from build123d import *

# Parameters (mm, degrees)
BOSS_EXTRUDE1_DEPTH  = 2
BOSS_EXTRUDE6_DEPTH  = 4.5
CUT_EXTRUDE6_DEPTH   = 4.5
BOSS_EXTRUDE14_DEPTH = 2.3
SKETCH32_R           = 2.1
CUT_EXTRUDE7_DEPTH   = 2.3
SKETCH33_W           = 12.5
SKETCH33_H           = 1.343145751
BOSS_EXTRUDE15_DEPTH = 1.2
SKETCH35_W           = 5.479645997
SKETCH35_H           = 3.827993755
CUT_EXTRUDE8_DEPTH   = 2.4
SKETCH36_W           = 3.7
SKETCH36_H           = 1.827993755
CUT_EXTRUDE9_DEPTH   = 2.4
SKETCH37_R           = 3.9
BOSS_EXTRUDE16_DEPTH = 4.4
CUT_EXTRUDE10_DEPTH  = 7.4
SKETCH43_R           = 2.5
BOSS_EXTRUDE17_DEPTH = 1.2
SKETCH44_R           = 0.95
CUT_EXTRUDE11_DEPTH  = 11
SKETCH45_R           = 2
CUT_EXTRUDE12_DEPTH  = 4.5
SKETCH52_R           = 0.75
CUT_EXTRUDE13_DEPTH  = 10


with BuildPart() as part:
    # Sketch3 → Boss-Extrude1 (new body)
    with BuildSketch(Plane.XY):
        with BuildLine():
            Line((8, 0), (9, -2.5))
            Line((9, -2.5), (9, -7))
            Line((9, -7), (21.5, -7))
            Line((21.5, -7), (25.050252532, -4.949747468))
            ThreePointArc((25.050252532, -4.949747468), (36.467156728, -2.678784027), (30, 7))
            Line((30, 7), (27, 7.5))
            Line((27, 7.5), (5.656854249, 7.5))
            Line((5.656854249, 7.5), (5.656854249, 5.656854249))
            ThreePointArc((5.656854249, 5.656854249), (7.39103626, 3.061467459), (8, 0))
        make_face()
    extrude(amount=BOSS_EXTRUDE1_DEPTH)

    # Sketch22 → Boss-Extrude6 (add)
    with BuildSketch(Plane.XY.offset(2)):
        with BuildLine():
            Line((5.656854249, 5.656854249), (2.486790148, 5.656854249))
            Line((2.486790148, 5.656854249), (2.486790148, 7.5))
            Line((2.486790148, 7.5), (5.656854249, 7.5))
            Line((5.656854249, 7.5), (21.5, 7.5))
            Line((21.5, 7.5), (27, 7.5))
            Line((27, 7.5), (27, 2.172006245))
            Line((27, 2.172006245), (23.275126266, 2.172006245))
            Line((23.275126266, 2.172006245), (23.275126266, -5.974873734))
            Line((23.275126266, -5.974873734), (21.5, -7))
            Line((21.5, -7), (9, -7))
            Line((9, -7), (9, -2.5))
            Line((9, -2.5), (8, 0))
            ThreePointArc((8, 0), (7.39103626, 3.061467459), (5.656854249, 5.656854249))
        make_face()
    extrude(amount=BOSS_EXTRUDE6_DEPTH)

    # Sketch26 → Cut-Extrude6 (cut)
    with BuildSketch(Plane.XY.offset(2)):
        Polygon((18.098080448, 5.3), (2.530052458, 5.3), (2.530052458, 4), (18.098080448, 4), (27, 4), (27, 5.3), align=None)
    extrude(amount=CUT_EXTRUDE6_DEPTH, mode=Mode.SUBTRACT)


with BuildPart() as body_2:
    # Sketch31 → Boss-Extrude14 (new body)
    with BuildSketch(Plane.XY.offset(6.5)):
        with BuildLine():
            Line((2.432688066, 5.656854249), (0, 5.656854249))
            ThreePointArc((0, 5.656854249), (-5.656854249, 0), (0, -5.656854249))
            Line((0, -5.656854249), (9, -5.656854249))
            Line((9, -5.656854249), (9, -7))
            Line((9, -7), (21.5, -7))
            Line((21.5, -7), (23.275126266, -5.974873734))
            Line((23.275126266, -5.974873734), (23.275126266, 2.172006245))
            Line((23.275126266, 2.172006245), (27, 2.172006245))
            Line((27, 2.172006245), (27, 7.5))
            Line((27, 7.5), (2.486790148, 7.5))
            Line((2.486790148, 7.5), (2.432688066, 5.656854249))
        make_face()
    extrude(amount=BOSS_EXTRUDE14_DEPTH)

    # Sketch32 → Cut-Extrude7 (cut)
    with BuildSketch(Plane.XY.offset(8.8)):
        Circle(SKETCH32_R)
    extrude(amount=-CUT_EXTRUDE7_DEPTH, mode=Mode.SUBTRACT)

    # Sketch33 → Boss-Extrude15 (add)
    with BuildSketch(Plane.XY.offset(8.8)):
        with Locations((15.25, -6.328427125)):
            Rectangle(SKETCH33_W, SKETCH33_H)
        Polygon((2.486790148, 7.5), (21.5, 7.5), (21.5, 5.656854249), (2.432688066, 5.656854249), align=None)
    extrude(amount=BOSS_EXTRUDE15_DEPTH)


with BuildPart() as cut_extrude8_tool:
    # Sketch35 → Cut-Extrude8 (new body)
    with BuildSketch(Plane.XY.offset(8.8)):
        with Locations((24.260177002, 4.086003123)):
            Rectangle(SKETCH35_W, SKETCH35_H)
    extrude(amount=-CUT_EXTRUDE8_DEPTH)


with BuildPart() as part_1:
    add(part.part)

    # Cut-Extrude8: cut by cut_extrude8_tool
    add(cut_extrude8_tool.part, mode=Mode.SUBTRACT)

    # Sketch36 → Cut-Extrude9 (cut)
    with BuildSketch(Plane.XY.offset(6.4)):
        with Locations((25.15, 3.086003123)):
            Rectangle(SKETCH36_W, SKETCH36_H)
    extrude(amount=-CUT_EXTRUDE9_DEPTH, mode=Mode.SUBTRACT)

    # Sketch37 → Boss-Extrude16 (add)
    with BuildSketch(Plane.XY.offset(2)):
        with Locations((30, 0)):
            Circle(SKETCH37_R)
    extrude(amount=BOSS_EXTRUDE16_DEPTH)

    # Sketch39 → Cut-Extrude10 (cut, through all)
    with BuildSketch(Plane.XY.offset(6.4)):
        with BuildLine():
            Line((29, 1.732050808), (29, -1.732050808))
            ThreePointArc((29, -1.732050808), (32, 0), (29, 1.732050808))
        make_face()
    extrude(amount=-CUT_EXTRUDE10_DEPTH, mode=Mode.SUBTRACT)


with BuildPart() as body_2_1:
    add(body_2.part)

    # Cut-Extrude8: cut by cut_extrude8_tool
    add(cut_extrude8_tool.part, mode=Mode.SUBTRACT)

    # Sketch43 → Boss-Extrude17 (add)
    with BuildSketch(Plane.XY.offset(8.8)):
        with Locations((11.5, 0)):
            Circle(SKETCH43_R)
        with Locations((18, 0)):
            Circle(SKETCH43_R)
    extrude(amount=BOSS_EXTRUDE17_DEPTH)


with BuildPart() as cut_extrude11_tool:
    # Sketch44 → Cut-Extrude11 (new body, through all)
    with BuildSketch(Plane.XY.offset(10)):
        with Locations((11.5, 0)):
            Circle(SKETCH44_R)
        with Locations((18, 0)):
            Circle(SKETCH44_R)
    extrude(amount=-CUT_EXTRUDE11_DEPTH)


with BuildPart() as part_2:
    add(part_1.part)

    # Cut-Extrude11: cut by cut_extrude11_tool
    add(cut_extrude11_tool.part, mode=Mode.SUBTRACT)

    # Sketch45 → Cut-Extrude12 (cut)
    with BuildSketch(Plane(origin=(0, 0, 0), x_dir=(-1, 0, 0), z_dir=(0, 0, -1))):
        with Locations((-11.5, 0)):
            Circle(SKETCH45_R)
        with Locations((-18, 0)):
            Circle(SKETCH45_R)
    extrude(amount=-CUT_EXTRUDE12_DEPTH, mode=Mode.SUBTRACT)


with BuildPart() as body_2_2:
    add(body_2_1.part)

    # Cut-Extrude11: cut by cut_extrude11_tool
    add(cut_extrude11_tool.part, mode=Mode.SUBTRACT)

    # Sketch52 → Cut-Extrude13 (cut, along a direction that is not the sketch's normal)
    with BuildSketch(Plane.XZ.offset(-5.656854249)):
        with Locations((18.235476819, 10)):
            Circle(SKETCH52_R)
    extrude(amount=-CUT_EXTRUDE13_DEPTH, dir=(0.640410196, -0.76803306, 0), mode=Mode.SUBTRACT)


solid = part_2.part
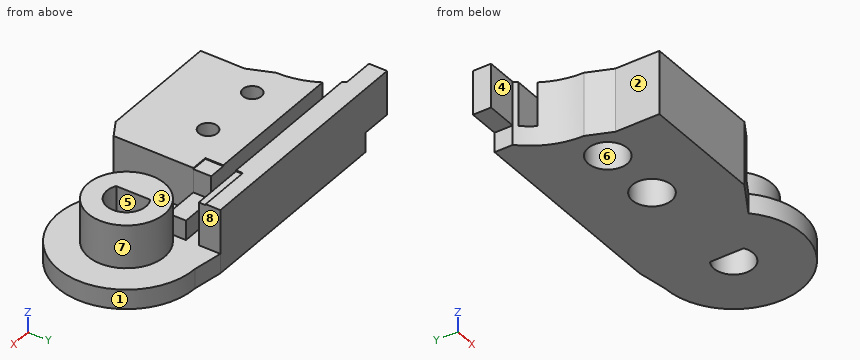
Design review of the part built by this model. Coordinates are the model's own, in mm. Face numbers are marked on the shaded views. A direction names the side the tool comes from. Give positions to 0.01 mm unless a question says otherwise; leave off trailing zeros. Order: outer loops, then holes, each group sorted by start corner. A loop starts at its lowest first (then second) coordinate and runs counter-clockwise, first axis right, second up. Notation, with made-up numbers: (-2.5, -30.75) - (8.5, -30.75) arc R31 ccw to (8.5, 0.25) - close; hole circle Ø11 at (46, 77). An arc over 180 degrees is marked (long way). Write item = value, one per line. Start each with the question number.
Q1. Mouldability with a two-part tool opening along X and no side actions: class the marked faces 1, 2 and 3 as released by +X, released by -X, zero draft, split by the parting line, or undercut.
Q2. We need section A-A on z = 5.75. State how many separate pieces and enclosed holes the cut face has, plus the area to 3 significant figures.
Q3. We need section B-B on x = 11.5. State the section outline as (y, z) points, plus the area to 3 significant figures.
Q4. Clearance check with flat-ended pins moving along their axes: pin 1 Ø1.5 at (y, z) = (1, 5.5) entering from -X; pin 2 Ø2 at (y, z) = (0, 1) entering from -X; pin 3 Ø1.2 at (x, y) = (17, -0.5) entering from -Z. State where each tip first meets the part, or that it passes through.
Q5. We need section D-D on x = 33. State the section outline as (y, z) points, plus the area to 3 significant figures.
Q6. Tool access review of the marked faces 4, 5, 6, 7 and 8: name each direction out of +Z, -Z, +X, -X, +Y, -Y from which nothing blocks a thin tool from reaching the whole face with its end or side.
Q7. To check wall thickness, follow L1, parallel to Y at x = 18, z = 5.15; L2, parallel to Y at x = 16.5, z = 6; L3, parallel to Y at x = 10.5, z = 3.25. State the ranges of each line that lie inside material, in increasing order. Write a range as from..to.
Q8. We need section C-C on z = 2.5. State the section outline as (x, y) points.
Working result:
q1.face_1 = undercut
q1.face_2 = released by -X
q1.face_3 = zero draft
q2.separate_pieces = 3
q2.enclosed_holes = 3
q2.area = 248 mm²
q3.outline = (-7, 0) - (-2, 0) - (-2, 4.5) - (-0.95, 4.5) - (-0.95, 6.5) - (-7, 6.5) - close; (0.95, 4.5) - (2, 4.5) - (2, 0) - (7.5, 0) - (7.5, 6.5) - (5.3, 6.5) - (5.3, 2) - (4, 2) - (4, 6.5) - (0.95, 6.5) - close
q3.area = 66.6 mm²
q4.pin_1 = 7.81
q4.pin_2 = 7.94
q4.pin_3 = 4.5
q5.outline = (-6.32, 0) - (6.32, 0) - (6.32, 2) - (2.49, 2) - (2.49, 6.4) - (-2.49, 6.4) - (-2.49, 2) - (-6.32, 2) - close
q5.area = 47.2 mm²
q6.face_4 = +Z, -Z, -X, -Y
q6.face_5 = +Z, -Z
q6.face_6 = -Z
q6.face_7 = +Z
q6.face_8 = +Z, +X, +Y
q7.L1 = -7..-0.95, 0.95..4, 5.3..7.5
q7.L2 = -7..4, 5.3..7.5
q7.L3 = -7..-1.73, 1.73..4, 5.3..7.5
q8.outline = (2.49, 5.66) - (5.66, 5.66) arc R8 cw to (5.99, 5.3) - (27, 5.3) - (27, 7.5) - (2.49, 7.5) - close; (6.93, 4) arc R8 cw to (8, 0) - (9, -2.5) - (9, -7) - (21.5, -7) - (23.28, -5.97) - (23.28, 2.17) - (26.76, 2.17) arc R3.9 ccw (long way) to (27, 2.49) - (27, 4) - close; hole circle Ø4 at (11.5, 0); hole circle Ø4 at (18, 0); hole (29, -1.73) arc R2 ccw (long way) to (29, 1.73) - close
